Geometry: final body of the model. Coordinates: model frame, mm. Coordinates: 2 decimals unless noted, no trailing zeros. Write each loop counter-clockwise with the first axis right and the second up, starting at its lowest first coordinate (ties: lowest second). Pieces come first, ordered by that corner, then holes. Notation, with made-up numbers: (0, 69.5) -> (10, 69.5) arc R36 cw to (10, 104.5) -> close; hole circle Ø1 at (82.25, -4.75). An arc over 180 degrees is marked (long way). One line per item, written item: value. Start each with the question number.
Autodesk Inventor part; units mm, degrees
ref_plane "YZ Plane" through (0, 0, 0) normal (1, 0, 0) x (0, 1, 0)
ref_plane "XZ Plane" through (0, 0, 0) normal (0, 1, 0) x (-1, 0, 0)
ref_plane "XY Plane" through (0, 0, 0) normal (0, 0, 1) x (1, 0, 0)
sketch "Эскиз1" plane through (0, 0, 0) normal (0, 0, 1) x (1, 0, 0)
  line L0 (0, 0) -> (48.5, 0)
  line L1 (48.5, 0) -> (48.5, -20)
  line L2 (48.5, -20) -> (6.9412, -20)
  line L3 (0, 0) -> (35, 0)
  line L4 (35, 0) -> (27.7206, -20)
  line L5 (0, -24) -> (0, 4)
  dimension "d0" = 48.5
  dimension "d1" = 20
  dimension "d2" = 35
  dimension "d3" = 70
revolve "Вращение1" add sketch "Эскиз1" angle 360 about axis through (0, -10, 0) along (0, 1, 0)
chamfer "Фаска1" distance 2 angle 45 2 edges at (-35, 0, 0) (-27.7206, -20, 0)
chamfer "Фаска2" distance 2 angle 45 2 edges at (-48.5, -20, 0) (-48.5, 0, 0)
properties part number "Кольцо поршень-шток верх_CPY" material "Сталь, мягкая"
Q1. Cut plane A-A on x = 0. Output: boundary loops of the cut face in (y, z).
Q2. Cut plane C-C on y = -14.75. Output: boundary loops of the cut face in (x, z), and give its area (3 significant figures).
Q3. Line query: L1, parallel to Z at x = 15, y = -1.5; L2, parallel to Z at x = 9, y = -8.25; L3, parallel to X at y = -17.75, z = 14.5. Output: solid intervals per line, ascending. Write a range as from..to.
Q4. First-contact query: P1, Ø3, axis at y = -16, z = 3.5, coming from the -X side; P2, Ø1, axis at x = -35, z = -37, coming from the +Y side; P3, Ø1, axis at x = 8, y = -16, coming from the -Z side; P4, Ø8, axis at x = -34, y = -13.5, coming from the +Z side. Flat tips, straight axial feed; report the tip coordinate or a pass-through.
Q5. Cut plane D-D on y = -7.75. Output: boundary loops of the cut face in (x, z).
Q6. Cut plane B-B on z = 0. Output: boundary loops of the cut face in (x, y).
Q7. Draft query along X for faces 1 (the flat face through (-31.2, 0, 20.4)), 2 (the conical face through (-7.475, -1.762, 33.664)), 3 (the conical face through (44.472, -0.125, 14.005)), 4 (the conical face through (-22.834, -17.105, 17.509)). Return one class per face: pulls with the +X half, pulls with the -X half, needs draft (parallel to the pull), parting line crosses it, or undercut.
Solution:
1. outline: (-20, -46.5) -> (-18, -48.5) -> (-2, -48.5) -> (0, -46.5) -> (0, -37) -> (-1.88, -34.32) -> (-18.12, -28.4) -> (-20, -29.72) -> close; (-20, 29.72) -> (-18.12, 28.4) -> (-1.88, 34.32) -> (0, 37) -> (0, 46.5) -> (-2, 48.5) -> (-18, 48.5) -> (-20, 46.5) -> close
2. outline: circle Ø97 at (0, 0); hole circle Ø59.26 at (0, 0)
2. area: 4,630 mm²
3. L1: -45.6..-31.47, 31.47..45.6
3. L2: -47.66..-30.71, 30.71..47.66
3. L3: -46.28..-24.58, 24.58..46.28
4. P1: x = -48.46
4. P2: through
4. P3: z = -47.92
4. P4: z = 38.11
5. outline: circle Ø97 at (0, 0); hole circle Ø64.36 at (0, 0)
6. outline: (-48.5, -18) -> (-46.5, -20) -> (-29.72, -20) -> (-28.4, -18.12) -> (-34.32, -1.88) -> (-37, 0) -> (-46.5, 0) -> (-48.5, -2) -> close; (28.4, -18.12) -> (29.72, -20) -> (46.5, -20) -> (48.5, -18) -> (48.5, -2) -> (46.5, 0) -> (37, 0) -> (34.32, -1.88) -> close
7. face 1: needs draft
7. face 2: undercut
7. face 3: parting line crosses it
7. face 4: undercut
